For this review, take the finished solid that the model builds, in its own axes (mm). Give positions to 0.01 mm unless a question says otherwise; leave off trailing zeros. Write each loop counter-clockwise with the first axis right and the second up, starting at its lowest first coordinate (ties: lowest second). Pieces come first, ordered by that corner, then holes. Notation, with made-up numbers: (17.5, 10.25) -> (69.5, 10.25) arc R13 ccw to (69.5, 21.25) -> close; hole circle Ø7 at (82, 59). An arc over 180 degrees is marked (long way). Write item = value, one per line.
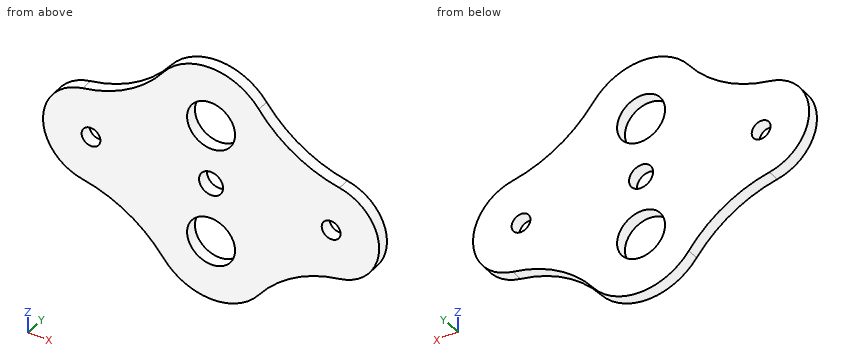
```python
from build123d import *

# Parameters (mm, degrees)
BOSS_EXTRUDE1_DEPTH         = 3.175
F_1_4_0_25_DIAMETER_HOLE1_D = 6.35
SKETCH5_R                   = 6.35
CUT_EXTRUDE1_DEPTH          = 4.175
SKETCH6_R                   = 2.4892
CUT_EXTRUDE2_DEPTH          = 4.175


with BuildPart() as part:
    # Sketch1 → Boss-Extrude1 (new body)
    with BuildSketch(Plane(origin=(0, 0, 0), x_dir=(1, 0, 0), z_dir=(0, 1, 0))):
        with BuildLine():
            ThreePointArc((12.62743016, 25.495999561), (0, 31.75), (-12.62743016, 25.495999561))
            ThreePointArc((-12.62743016, 25.495999561), (-22.066120108, 16.991504417), (-33.953426839, 12.50739422))
            ThreePointArc((-33.953426839, 12.50739422), (-44.45, 0), (-33.953426839, -12.50739422))
            ThreePointArc((-33.953426839, -12.50739422), (-22.066120108, -16.991504417), (-12.62743016, -25.495999561))
            ThreePointArc((-12.62743016, -25.495999561), (0, -31.75), (12.62743016, -25.495999561))
            ThreePointArc((12.62743016, -25.495999561), (22.066120108, -16.991504417), (33.953426839, -12.50739422))
            ThreePointArc((33.953426839, -12.50739422), (44.45, 0), (33.953426839, 12.50739422))
            ThreePointArc((33.953426839, 12.50739422), (22.066120108, 16.991504417), (12.62743016, 25.495999561))
        make_face()
    extrude(amount=BOSS_EXTRUDE1_DEPTH)

    # 1/4 (0.25) Diameter Hole1 (through all)
    with Locations(Plane(origin=(0, 3.175, 0), x_dir=(1, 0, 0), z_dir=(0, 1, 0))):
        with Locations((0, 0)):
            Hole(F_1_4_0_25_DIAMETER_HOLE1_D / 2)

    # Sketch5 → Cut-Extrude1 (cut, through all)
    with BuildSketch(Plane(origin=(0, 3.175, 0), x_dir=(1, 0, 0), z_dir=(0, 1, 0))):
        with Locations((0, 15.875)):
            Circle(SKETCH5_R)
        with Locations((0, -15.875)):
            Circle(SKETCH5_R)
    extrude(amount=-CUT_EXTRUDE1_DEPTH, mode=Mode.SUBTRACT)

    # Sketch6 → Cut-Extrude2 (cut, through all)
    with BuildSketch(Plane(origin=(0, 3.175, 0), x_dir=(1, 0, 0), z_dir=(0, 1, 0))):
        with Locations((-31.75, 0)):
            Circle(SKETCH6_R)
        with Locations((31.75, 0)):
            Circle(SKETCH6_R)
    extrude(amount=-CUT_EXTRUDE2_DEPTH, mode=Mode.SUBTRACT)


solid = part.part
```
(1) For pin 1 (1 mm diameter, centred on x = -34.5, y = 1.5, fed in from -Z), flat-tipped, find the tip position at first contact; note if it passes through.
Answers below:
pin_1 = -12.5
(2) Take a section at C-C (z = -14.5). Write out the cut boundary in (x, y) (3 decimals).
Answers below:
outline = (-27.018, 0) -> (-6.199, 0) -> (-6.199, 3.175) -> (-27.018, 3.175) -> close; (6.199, 0) -> (27.018, 0) -> (27.018, 3.175) -> (6.199, 3.175) -> close
(3) Take a section at D-D (x = 31.75). Write out the cut boundary in (y, z) (3 decimals).
Answers below:
outline = (0, -12.971) -> (3.175, -12.971) -> (3.175, -2.489) -> (0, -2.489) -> close; (0, 2.489) -> (3.175, 2.489) -> (3.175, 12.971) -> (0, 12.971) -> close
(4) To check wall thickness, follow probe 1 along Z at (x, y) = (4, 2.95); probe 2 along Z at (x, y) = (1.5, 1.15); probe 3 along Z at (x, y) = (31.75, 0.7). State the ranges of each line that lie inside material, in increasing order.
Answers below:
probe_1 = -31.24 to -20.81, -10.94 to 10.94, 20.81 to 31.24
probe_2 = -31.68 to -22.05, -9.7 to -2.8, 2.8 to 9.7, 22.05 to 31.68
probe_3 = -12.97 to -2.49, 2.49 to 12.97
(5) Take a section at B-B (z = 0). Write out the cut boundary in (x, y) (3 decimals).
Answers below:
outline = (-44.45, 0) -> (-34.239, 0) -> (-34.239, 3.175) -> (-44.45, 3.175) -> close; (-29.261, 0) -> (-3.175, 0) -> (-3.175, 3.175) -> (-29.261, 3.175) -> close; (3.175, 0) -> (29.261, 0) -> (29.261, 3.175) -> (3.175, 3.175) -> close; (34.239, 0) -> (44.45, 0) -> (44.45, 3.175) -> (34.239, 3.175) -> close
(6) Take a section at A-A (x = 0). Write out the cut boundary in (y, z) (3 decimals), plus the area to 3 significant figures.
Answers below:
outline = (0, -31.75) -> (3.175, -31.75) -> (3.175, -22.225) -> (0, -22.225) -> close; (0, -9.525) -> (3.175, -9.525) -> (3.175, -3.175) -> (0, -3.175) -> close; (0, 3.175) -> (3.175, 3.175) -> (3.175, 9.525) -> (0, 9.525) -> close; (0, 22.225) -> (3.175, 22.225) -> (3.175, 31.75) -> (0, 31.75) -> close
area = 101 mm^2
